```python
from build123d import *

# Parameters (mm, degrees)
CUT_EXTRUDE1_DEPTH      = 111.145358504
CUT_EXTRUDE1_DEPTH_BACK = 111.145358504
SKETCH2_R               = 6
SKETCH5_W               = 12
SKETCH5_H               = 8.82137068
CUT_EXTRUDE3_DEPTH      = 6


with BuildPart() as part:
    # Sketch1 → Revolve1 (revolve)
    with BuildSketch(Plane(origin=(0, 0, 0), x_dir=(1, 0, 0), z_dir=(0, 1, 0))):
        Polygon((24, 78), (24, 72), (34, 72), (34, 42), (30, 42), (30, 0), (40, 4), (40, 32), (72, 32), (72, 42), (40, 42), (40, 72), (34, 78), align=None)
    revolve(axis=Axis((0, 0, 0), (0, 0, -1)))

    # Sketch2 → Cut-Extrude1 (cut, two sides: drawn at the far end of the back side and taken through both)
    with BuildSketch(Plane(origin=(0, 0, -42), x_dir=(-1, 0, 0), z_dir=(0, 0, -1)).offset(-CUT_EXTRUDE1_DEPTH_BACK)):
        with Locations((0, 58)):
            Circle(SKETCH2_R)
        with Locations((58, 0)):
            Circle(SKETCH2_R)
        with Locations((0, -58)):
            Circle(SKETCH2_R)
        with Locations((-58, 0)):
            Circle(SKETCH2_R)
    extrude(amount=CUT_EXTRUDE1_DEPTH + CUT_EXTRUDE1_DEPTH_BACK, mode=Mode.SUBTRACT)

    # Sketch5 → Cut-Extrude3 (cut)
    with BuildSketch(Plane.XY):
        with Locations((0, 30)):
            Rectangle(SKETCH5_W, SKETCH5_H)
        with Locations((0, -30)):
            Rectangle(SKETCH5_W, SKETCH5_H)
    extrude(amount=-CUT_EXTRUDE3_DEPTH, mode=Mode.SUBTRACT)


solid = part.part
```
Source: CAD feature listing. Evaluate the final solid. Frame: model axes, mm. A direction names the side the tool comes from. Give positions to 0.01 mm unless a question says otherwise; leave off trailing zeros. Write each loop counter-clockwise with the first axis right and the second up, starting at its lowest first coordinate (ties: lowest second). Pieces come first, ordered by that corner, then holes.
1. Section query C-C (y = -58). Return the cut outline in (x, z), then the cut area to 3 significant figures.
2. Access query for faces 1 (the face through (18.28, -28.67, -56.79)), 2 (the face through (-8.67, 39.05, -18.2)), 3 (the face through (31, 31, -42)). Directions: +Z, -Z, +X, -X, +Y, -Y. A direction counts if a zero-diameter tool reaches every point of the face in a straight line with its end or side. Return the directions, or none.
3. Pull-direction query (Z, two-part tool) for faces 4 (the face through (7.1, -23.1, -78)), 5 (the face through (2.4, 30.1, -42)), 6 (the face through (-8.67, 39.05, -57.21)); classes: +Z half, -Z half, draft (parallel to the pull), parting line (faces both ways), or undercut.
4. First-contact query: pin 1 (1.5 mm diameter, centred on y = -9, z = -44.5, fed in from -X); pin 2 (10 mm diameter, centred on x = 36, z = -20.5, fed in from -Y); pin 3 (5.5 mm diameter, centred on y = 33, z = -2.5, fed in from -X); pin 4 (11 mm diameter, centred on x = 58, y = 0, fed in from -Z). Flat tips, straight axial feed; report the tip coordinate or a pass-through.
5. Material intervals for line 1 along X through (y, z) = (0, -36.75); line 2 along Y through (x, z) = (1, -61.5), sorted ascending.
6. Section query B-B (y = 0). Count the separate pieces of the cut face and the enclosed holes in it, then the cut area to 3 significant figures.
7. Section query A-A (x = -61). Return the cut outline in (y, z), then the cut area to 3 significant figures.
Output values:
1. outline: (-42.66, -42) - (-6, -42) - (-6, -32) - (-42.66, -32) - close; (6, -42) - (42.66, -42) - (42.66, -32) - (6, -32) - close
1. area: 733 mm2
2. face 1: none
2. face 2: +Z
2. face 3: -Z
3. face 4: -Z half
3. face 5: undercut
3. face 6: draft
4. pin 1: stops at x = -39.14
4. pin 2: stops at y = -25.28
4. pin 3: stops at x = -25.65
4. pin 4: passes through
5. line 1: x = -72 to -64, -52 to -30, 30 to 52, 64 to 72
5. line 2: y = -39.99 to -33.99, 33.99 to 39.99
6. separate pieces: 4
6. enclosed holes: 0
6. area: 1,720 mm2
7. outline: (-38.25, -42) - (-5.2, -42) - (-5.2, -32) - (-38.25, -32) - close; (5.2, -42) - (38.25, -42) - (38.25, -32) - (5.2, -32) - close
7. area: 661 mm2
